from build123d import *

# Parameters (mm, degrees)
F0_W     = 278
F0_H     = 400
F1_DEPTH = 110
F2_W     = 258
F2_H     = 380
F3_DEPTH = 100
F4_W     = 400
F4_H     = 20
F5_DEPTH = 15
F6_W     = 400
F6_H     = 20
F7_DEPTH = 15


with BuildPart() as f1:
    # F0 (on Top) → F1 (new body)
    with BuildSketch(Plane.XY):
        Rectangle(F0_W, F0_H)
    extrude(amount=F1_DEPTH)

    # F2 (on face) → F3 (cut)
    with BuildSketch(Plane.XY.offset(110)):
        Rectangle(F2_W, F2_H)
    extrude(amount=-F3_DEPTH, mode=Mode.SUBTRACT)

    # F4 (on face) → F5 (join)
    with BuildSketch(Plane(origin=(-139, 0, 0), x_dir=(0, -1, 0), z_dir=(-1, 0, 0))):
        with Locations((0, 75)):
            Rectangle(F4_W, F4_H)
    extrude(amount=F5_DEPTH)

    # F6 (on face) → F7 (join)
    with BuildSketch(Plane.YZ.offset(139)):
        with Locations((0, 75)):
            Rectangle(F6_W, F6_H)
    extrude(amount=F7_DEPTH)


solid = f1.part
For this review, take the finished solid that the model builds, in its own axes (mm). A direction names the side the tool comes from. Give positions to 0.01 mm unless a question says otherwise; leave off trailing zeros. Write each loop counter-clockwise with the first axis right and the second up, starting at its lowest first coordinate (ties: lowest second). Pieces come first, ordered by that corner, then holes. Notation, with made-up numbers: (88, 6.25) -> (144, 6.25) arc R34 ccw to (144, 39.25) -> close; hole circle Ø7 at (-37, 76.5). An arc over 180 degrees is marked (long way). Use CSV: the item, a comma, the result in double quotes.
Q1. To check wall thickness, follow probe 1 along X at (y, z) = (165.5, 90.5); probe 2 along Y at (x, z) = (-60, 36.5); probe 3 along X at (y, z) = (101, 80.5). State the ranges of each line that lie inside material, in increasing order. Write a range as [from, to].
Conclusion:
probe 1,"[-139, -129], [129, 139]"
probe 2,"[-200, -190], [190, 200]"
probe 3,"[-154, -129], [129, 154]"
Q2. Take a section at C-C, the plane x = 23. Write out the cut boundary in (y, z).
Conclusion:
outline,"(-200, 0) -> (200, 0) -> (200, 110) -> (190, 110) -> (190, 10) -> (-190, 10) -> (-190, 110) -> (-200, 110) -> close"
Q3. Tool access review of faces 1 (the face through (-146, 3, 85)), 2 (the face through (139, -3, 32)), 3 (the face through (139, -3, 97)): name each direction out of +Z, -Z, +X, -X, +Y, -Y from which nothing blocks a thin tool from reaching the whole face with its end or side.
Conclusion:
face 1,"+Z, -X, +Y, -Y"
face 2,"-Z, +X, +Y, -Y"
face 3,"+Z, +X, +Y, -Y"
Q4. Take a section at A-A, the plane z = 56. Write out the cut boundary in (x, y).
Conclusion:
outline,"(-139, -200) -> (139, -200) -> (139, 200) -> (-139, 200) -> close; hole (-129, -190) -> (129, -190) -> (129, 190) -> (-129, 190) -> close"
Q5. Take a section at B-B, the plane y = 147. Write out the cut boundary in (x, z), then the cut area to 3 significant figures.
Conclusion:
outline,"(-154, 65) -> (-139, 65) -> (-139, 0) -> (139, 0) -> (139, 65) -> (154, 65) -> (154, 85) -> (139, 85) -> (139, 110) -> (129, 110) -> (129, 10) -> (-129, 10) -> (-129, 110) -> (-139, 110) -> (-139, 85) -> (-154, 85) -> close"
area,"5,380 mm2"
Q6. For P1, Ø12, axis at x = -149, y = -86.5, coming from the +Z side; P2, Ø19.5, axis at y = -68.5, z = 44, coming from the -X side; P3, Ø1.5, axis at x = 13.5, y = 79, coming from the +Z side; P4, Ø2, axis at x = -18.5, y = -47.5, coming from the -Z side, all flat-tipped, find the tip position at first contact; note any pin that passes through.
Conclusion:
P1,"z = 85"
P2,"x = -139"
P3,"z = 10"
P4,"z = 0"
Q7. Mouldability with a two-part tool opening along Y and no side actions: class faces 4 (the face through (146, -3, 85)), 5 (the face through (-2, 3, 10)), 6 (the face through (-2, 200, 54)) as pulls with the +Y half, pulls with the -Y half, needs draft (parallel to the pull), parting line crosses it, or undercut.
Conclusion:
face 4,"needs draft"
face 5,"undercut"
face 6,"pulls with the +Y half"
